```python
from build123d import *

# Parameters (mm, degrees)
SKETCH1_W           = 38.62
SKETCH1_H           = 24.72
SKETCH1_R           = 2.11
BOSS_EXTRUDE1_DEPTH = 1.3
SKETCH2_W           = 38.62
SKETCH2_H           = 13.7
BOSS_EXTRUDE2_DEPTH = 1.3


with BuildPart() as part:
    # Sketch1 → Boss-Extrude1 (new body)
    with BuildSketch(Plane.XY):
        with Locations((-21.272112536, 4.996529857)):
            Rectangle(SKETCH1_W, SKETCH1_H)
        with Locations((-33.952112536, 10.926529857)):
            Circle(SKETCH1_R, mode=Mode.SUBTRACT)
        with Locations((-21.272112536, 10.926529857)):
            Circle(SKETCH1_R, mode=Mode.SUBTRACT)
        with Locations((-8.592112536, 10.926529857)):
            Circle(SKETCH1_R, mode=Mode.SUBTRACT)
        with Locations((-21.272112536, -1.753470143)):
            Circle(SKETCH1_R, mode=Mode.SUBTRACT)
        with Locations((-8.592112536, -1.753470143)):
            Circle(SKETCH1_R, mode=Mode.SUBTRACT)
        with Locations((-33.952112536, -1.753470143)):
            Circle(SKETCH1_R, mode=Mode.SUBTRACT)
    extrude(amount=-BOSS_EXTRUDE1_DEPTH)

    # Sketch2 → Boss-Extrude2 (add)
    with BuildSketch(Plane.XZ.offset(7.363470143)):
        with Locations((-21.272112536, -6.85)):
            Rectangle(SKETCH2_W, SKETCH2_H)
        with BuildLine():
            Line((-31.842112536, -4.791404459), (-31.842112536, -9.091404459))
            ThreePointArc((-31.842112536, -9.091404459), (-33.952112536, -11.201404459), (-36.062112536, -9.091404459))
            Line((-36.062112536, -9.091404459), (-36.062112536, -4.791404459))
            ThreePointArc((-36.062112536, -4.791404459), (-33.952112536, -2.681404459), (-31.842112536, -4.791404459))
        make_face(mode=Mode.SUBTRACT)
        with BuildLine():
            Line((-19.162112536, -4.791404459), (-19.162112536, -9.091404459))
            ThreePointArc((-19.162112536, -9.091404459), (-21.272112536, -11.201404459), (-23.382112536, -9.091404459))
            Line((-23.382112536, -9.091404459), (-23.382112536, -4.791404459))
            ThreePointArc((-23.382112536, -4.791404459), (-21.272112536, -2.681404459), (-19.162112536, -4.791404459))
        make_face(mode=Mode.SUBTRACT)
        with BuildLine():
            Line((-6.482112536, -4.791404459), (-6.482112536, -9.091404459))
            ThreePointArc((-6.482112536, -9.091404459), (-8.592112536, -11.201404459), (-10.702112536, -9.091404459))
            Line((-10.702112536, -9.091404459), (-10.702112536, -4.791404459))
            ThreePointArc((-10.702112536, -4.791404459), (-8.592112536, -2.681404459), (-6.482112536, -4.791404459))
        make_face(mode=Mode.SUBTRACT)
    extrude(amount=-BOSS_EXTRUDE2_DEPTH)


solid = part.part
```
Can you work these out from the model? Positions are in its coordinate system, mm. A direction names the side the tool comes from. Coordinates: 2 decimals unless noted, no trailing zeros. Write each loop counter-clockwise with the first axis right and the second up, starting at its lowest first coordinate (ties: lowest second). Pieces come first, ordered by that corner, then holes. Notation, with made-up numbers: (-2, 18.5) - (44, 18.5) arc R28 cw to (44, 36.5) - close; hole circle Ø6 at (-10, 15). An arc over 180 degrees is marked (long way). Return JSON: item names as keys, results as strings.
Q1. If we section it at A-A (z = -7.5): Please give me the cut outline in (x, y).
Computed values:
{"outline": "(-40.58, -7.36) - (-36.06, -7.36) - (-36.06, -6.06) - (-40.58, -6.06) - close; (-31.84, -7.36) - (-23.38, -7.36) - (-23.38, -6.06) - (-31.84, -6.06) - close; (-19.16, -7.36) - (-10.7, -7.36) - (-10.7, -6.06) - (-19.16, -6.06) - close; (-6.48, -7.36) - (-1.96, -7.36) - (-1.96, -6.06) - (-6.48, -6.06) - close"}
Q2. On a 3-axis mill with a long thin cutter (end or side, diameter ignored), from which of +Z, -Z, +X, -X, +Y, -Y can I reach the whole of each face in a straight line? I mean faces 5 (the cylindrical face through (-10.1, 12.4, -0.6)), 6 (the flat face through (-22, -6.063, -12)), 7 (the cylindrical face through (-33.9, -6.7, -11.2)). Say none if no direction works.
Computed values:
{"face 5": "+Z, -Z", "face 6": "-Z, +X, -X, +Y", "face 7": "+Y, -Y"}
Q3. If we section it at B-B (x = -9.5): Please give me the cut outline in (y, z), then the cut area to 3 significant figures.
Computed values:
{"outline": "(-7.36, -13.7) - (-6.06, -13.7) - (-6.06, -11) - (-7.36, -11) - close; (-7.36, -2.89) - (-6.06, -2.89) - (-6.06, -1.3) - (-3.66, -1.3) - (-3.66, 0) - (-7.36, 0) - close; (0.15, -1.3) - (9.02, -1.3) - (9.02, 0) - (0.15, 0) - close; (12.83, -1.3) - (17.36, -1.3) - (17.36, 0) - (12.83, 0) - close", "area": "27.8 mm2"}
Q4. I'm going to push a flat-ended pin straight in: pin 1 Ø5 at (x, y) = (-29, -3.5) entering from -Z. Where does the tip first touch, or does it pass through?
Computed values:
{"pin 1": "stops at z = -1.3"}
Q5. Please list where these lines run through material, in increasing order: L1, parallel to Y at x = -15, z = -5.5; L2, parallel to Z at x = -14, y = 13.25. Write a range as from..to.
Computed values:
{"L1": "y = -7.36..-6.06", "L2": "z = -1.3..0"}
Q6. If we section it at D-D (x = -4.5): Please give me the cut outline in (y, z), then the cut area to 3 significant figures.
Computed values:
{"outline": "(-7.36, -13.7) - (-6.06, -13.7) - (-6.06, -1.3) - (17.36, -1.3) - (17.36, 0) - (-7.36, 0) - close", "area": "48.3 mm2"}
Q7. If we section it at C-C (y = -0.75): Please give me the cut outline in (x, z).
Computed values:
{"outline": "(-40.58, -1.3) - (-35.81, -1.3) - (-35.81, 0) - (-40.58, 0) - close; (-32.1, -1.3) - (-23.13, -1.3) - (-23.13, 0) - (-32.1, 0) - close; (-19.42, -1.3) - (-10.45, -1.3) - (-10.45, 0) - (-19.42, 0) - close; (-6.74, -1.3) - (-1.96, -1.3) - (-1.96, 0) - (-6.74, 0) - close"}
Q8. Thinking about a two-plate mould opening in Z: for faces 1 (the flat face through (-22, 5, 0)), 2 (the flat face through (-23.382, -7, -7)), 3 (the cylindrical face through (-10.7, -1.7, -0.6)), 4 (the flat face through (-22, -7, -13.7)), which applies, +Z half, -Z half, draft (parallel to the pull), parting line (faces both ways), or undercut?
Computed values:
{"face 1": "+Z half", "face 2": "undercut", "face 3": "draft", "face 4": "-Z half"}
